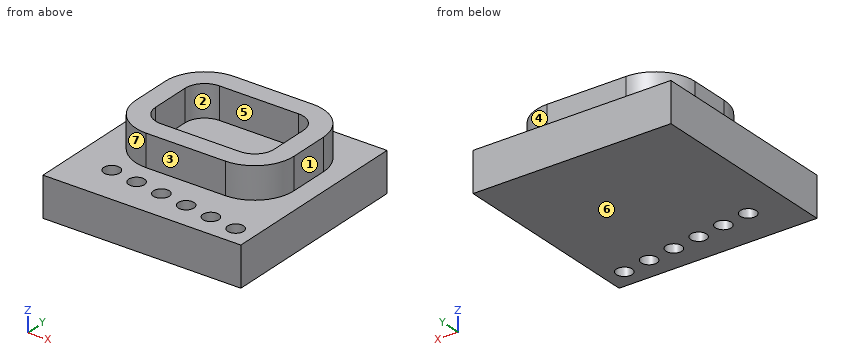
from build123d import *

# Parameters (mm, degrees)
F0_W     = 50
F0_H     = 50
F1_DEPTH = 10
F3_DEPTH = 8
F4_R     = 2.026375
F4_R_2   = 2
F5_DEPTH = 25


with BuildPart() as f1:
    # F0 (on Top) → F1 (new body)
    with BuildSketch(Plane.XY):
        with Locations((25, 25)):
            Rectangle(F0_W, F0_H)
    extrude(amount=F1_DEPTH)

    # F2 (on face) → F3 (join)
    with BuildSketch(Plane.XY.offset(10)):
        with BuildLine():
            Line((35, 45), (15, 45))
            ThreePointArc((15, 45), (7.928932, 42.071068), (5, 35))
            Line((5, 35), (5, 25))
            ThreePointArc((5, 25), (7.928932, 17.928932), (15, 15))
            Line((15, 15), (35, 15))
            ThreePointArc((35, 15), (42.071068, 17.928932), (45, 25))
            Line((45, 25), (45, 35))
            ThreePointArc((45, 35), (42.071068, 42.071068), (35, 45))
        make_face()
        with BuildLine():
            ThreePointArc((10, 35), (11.464466, 38.535534), (15, 40))
            Line((15, 40), (35, 40))
            ThreePointArc((35, 40), (38.535534, 38.535534), (40, 35))
            Line((40, 35), (40, 25))
            ThreePointArc((40, 25), (38.535534, 21.464466), (35, 20))
            Line((35, 20), (15, 20))
            ThreePointArc((15, 20), (11.464466, 21.464466), (10, 25))
            Line((10, 25), (10, 35))
        make_face(mode=Mode.SUBTRACT)
    extrude(amount=F3_DEPTH)

    # F4 (on face) → F5 (cut)
    with BuildSketch(Plane.XY.offset(10)):
        with Locations((10, 10)):
            Circle(F4_R)
        with Locations((17, 9)):
            Circle(F4_R_2)
        with Locations((24, 8)):
            Circle(F4_R_2)
        with Locations((31, 7)):
            Circle(F4_R_2)
        with Locations((38, 6)):
            Circle(F4_R_2)
        with Locations((45, 5)):
            Circle(F4_R_2)
    extrude(amount=-F5_DEPTH, mode=Mode.SUBTRACT)


solid = f1.part
Design review of the part built by this model. Coordinates are the model's own, in mm. Face numbers are marked on the shaded views. A direction names the side the tool comes from. Give positions to 0.01 mm unless a question says otherwise; leave off trailing zeros. Order: outer loops, then holes, each group sorted by start corner. A loop starts at its lowest first (then second) coordinate and runs counter-clockwise, first axis right, second up. Notation, with made-up numbers: (39.25, 49) - (51.25, 49) arc R13 cw to (51.25, 56) - close; hole circle Ø2 at (-31.5, 71.25). An arc over 180 degrees is marked (long way). Write item = value, one per line. Start each with the question number.
Q1. Tool access review of the marked faces 1, 2, 3 and 4: name each direction out of +Z, -Z, +X, -X, +Y, -Y from which nothing blocks a thin tool from reaching the whole face with its end or side.
Q2. We need section D-D on y = 31.5. State the section outline as (x, z) points.
Q3. We need section A-A on z = 1.75. State the section outline as (x, y) points.
Q4. Clearance check with flat-ended pins moving along their axes: pin 1 Ø10 at (y, z) = (38, 13) entering from -X; pin 2 Ø6.5 at (x, z) = (27.5, 15) entering from +Y; pin 3 Ø2.5 at (x, z) = (27, 15) entering from -Y; pin 4 Ø2.5 at (y, z) = (29, 14) entering from +X. State where each tip first meets the part, or that it passes through.
Q5. We need section C-C on z = 13. State the section outline as (x, y) points.
Q6. We need section B-B on x = 38. State the section outline as (y, z) points.
Q7. To check wall thickness, follow L1, parallel to Y at x = 31, z = 5.25; L2, parallel to Y at x = 45, z = 2.5; L3, parallel to Z at x = 20.5, y = 5. State the ranges of each line that lie inside material, in increasing order. Write a range as from..to.
Q8. Mouldability with a two-part tool opening along Y and no side actions: class the marked faces 5, 6 and 7 as released by +Y, released by -Y, zero draft, split by the parting line, or undercut.
Working result:
q1.face_1 = +Z, +X, +Y, -Y
q1.face_2 = +Z
q1.face_3 = +Z, +X, -X, -Y
q1.face_4 = +Z, +X, +Y
q2.outline = (0, 0) - (50, 0) - (50, 10) - (45, 10) - (45, 18) - (40, 18) - (40, 10) - (10, 10) - (10, 18) - (5, 18) - (5, 10) - (0, 10) - close
q3.outline = (0, 0) - (50, 0) - (50, 50) - (0, 50) - close; hole circle Ø4.05 at (10, 10); hole circle Ø4 at (17, 9); hole circle Ø4 at (24, 8); hole circle Ø4 at (31, 7); hole circle Ø4 at (38, 6); hole circle Ø4 at (45, 5)
q4.pin_1 = 0
q4.pin_2 = 45
q4.pin_3 = 15
q4.pin_4 = 45
q5.outline = (5, 25) arc R10 ccw to (15, 15) - (35, 15) arc R10 ccw to (45, 25) - (45, 35) arc R10 ccw to (35, 45) - (15, 45) arc R10 ccw to (5, 35) - close; hole (10, 25) arc R5 ccw to (15, 20) - (35, 20) arc R5 ccw to (40, 25) - (40, 35) arc R5 ccw to (35, 40) - (15, 40) arc R5 ccw to (10, 35) - close
q6.outline = (0, 0) - (4, 0) - (4, 10) - (0, 10) - close; (8, 0) - (50, 0) - (50, 10) - (44.54, 10) - (44.54, 18) - (39, 18) - (39, 10) - (21, 10) - (21, 18) - (15.46, 18) - (15.46, 10) - (8, 10) - close
q7.L1 = 0..5, 9..50
q7.L2 = 0..3, 7..50
q7.L3 = 0..10
q8.face_5 = undercut
q8.face_6 = zero draft
q8.face_7 = released by -Y
